Work out the finished part from the listing and answer in its coordinate system (mm). Face numbers are marked on the shaded views. A direction names the side the tool comes from. Round coordinates to 2 decimals unless told otherwise and drop trailing zeros. Order: outer loops, then holes, each group sorted by start corner. A loop starts at its lowest first (then second) coordinate and runs counter-clockwise, first axis right, second up. Notation, with made-up numbers: (-22, 72.25) - (28, 72.25) arc R19 cw to (28, 101.25) - close; hole circle Ø6 at (44.25, 3.5). An arc over 180 degrees is marked (long way). Answer in a Markdown table with one row per item.
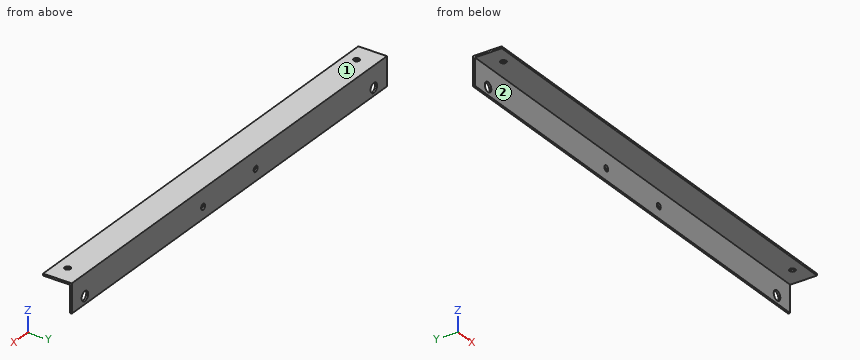
from build123d import *

# Parameters (mm, degrees)
EXTRU_MINCE1_DEPTH      = 120
ESQUISSE2_R             = 1.5
ENL_V_MAT_EXTRU_1_DEPTH = 3
ESQUISSE3_R             = 2.5
ESQUISSE3_R_2           = 1.5
ENL_V_MAT_EXTRU_2_DEPTH = 3


with BuildPart() as part:
    # Esquisse1 → Extru.-Mince1 (new, symmetric)
    with BuildSketch(Plane(origin=(0, 0, 0), x_dir=(0, 0, -1), z_dir=(1, 0, 0))):
        Polygon((0, -15), (0, 0), (15, 0), (15, -1), (1, -1), (1, -15), align=None)
    extrude(amount=EXTRU_MINCE1_DEPTH, both=True)

    # Esquisse2 → Enlèv. mat.-Extru.1 (cut)
    with BuildSketch(Plane.XY):
        with Locations((-110, -9)):
            Circle(ESQUISSE2_R)
        with Locations((110, -9)):
            Circle(ESQUISSE2_R)
    extrude(amount=-ENL_V_MAT_EXTRU_1_DEPTH, mode=Mode.SUBTRACT)

    # Esquisse3 → Enlèv. mat.-Extru.2 (cut)
    with BuildSketch(Plane(origin=(0, 0, 0), x_dir=(1, 0, 0), z_dir=(0, 1, 0))):
        with Locations(Location((-110, 11, 0), (0, 0, 270))):
            Circle(ESQUISSE3_R)
        with Locations(Location((-20, 9, 0), (0, 0, 270))):
            Circle(ESQUISSE3_R_2)
        with Locations(Location((110, 11, 0), (0, 0, 270))):
            Circle(ESQUISSE3_R)
        with Locations(Location((20, 9, 0), (0, 0, 270))):
            Circle(ESQUISSE3_R_2)
    extrude(amount=-ENL_V_MAT_EXTRU_2_DEPTH, mode=Mode.SUBTRACT)


solid = part.part
1) Find the intervals of material crossed by probe 1 along X at (y, z) = (-0.55, -11); probe 2 along X at (y, z) = (-0.5, -9); probe 3 along Y at (x, z) = (110, -0.7), in increasing order. Write a range as from..to.
Filled in:
| item | result |
|---|---|
| probe 1 | x = -120..-112.5, -107.5..107.5, 112.5..120 |
| probe 2 | x = -120..-111.5, -108.5..-21.5, -18.5..18.5, 21.5..108.5, 111.5..120 |
| probe 3 | y = -15..-10.5, -7.5..0 |
2) Find section B-B, the plane z = -3. Give the vertices of the cut face in (x, y), then the cut area to 3 significant figures.
Filled in:
| item | result |
|---|---|
| outline | (-120, -1) - (120, -1) - (120, 0) - (-120, 0) - close |
| area | 240 mm^2 |
3) Each of these flat-tipped pins is pushed along its axis until it touches: pin 1 (5 mm diameter, centred on x = -94.5, y = -12.5, fed in from -Z); pin 2 (8 mm diameter, centred on x = -85.5, y = -11.5, fed in from +Z); pin 3 (4 mm diameter, centred on x = -49.5, z = -8, fed in from -Y). Where does it stop, or does it pass through?
Filled in:
| item | result |
|---|---|
| pin 1 | stops at z = -1 |
| pin 2 | stops at z = 0 |
| pin 3 | stops at y = -1 |
4) Find section A-A, the plane x = -28. Give the vertices of the cut face in (y, z).
Filled in:
| item | result |
|---|---|
| outline | (-15, -1) - (-1, -1) - (-1, -15) - (0, -15) - (0, 0) - (-15, 0) - close |
5) Which of the six approach directions +Z, -Z, +X, -X, +Y, -Y give full straight-line access (tool end or side, diameter ignored) to the marked faces 1 and 2?
Filled in:
| item | result |
|---|---|
| face 1 | +Z, +X, -X, +Y, -Y |
| face 2 | -Z, +X, -X, -Y |
